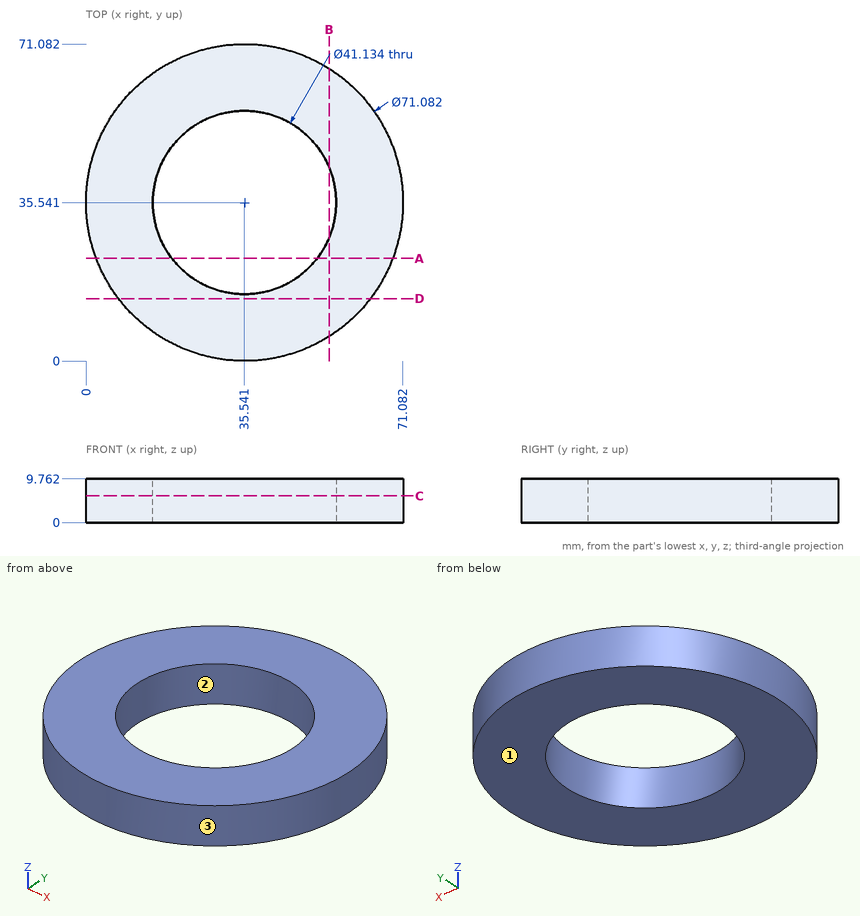
Here's the drawing with two shaded views (mm, measured from the low corner). I have some questions. Coordinates: 2 decimals unless noted, no trailing zeros. Loops run counter-clockwise (first coordinate to the right, second up) from the corner with the lowest first, then second, coordinate; pieces in that order, holes last. Notation, with made-up numbers: M 38.25,31 L 48.25,31 A21 ccw 48.25,41 Z; hole C -25.5,-14.75 d2. An arc over 180 degrees is marked long. Answer as CSV lines item,"result". Start each with the question number.
1. Suppose I cut it at A-A, the plane y = 23. List the corners of the cut face in (x, z) for me, plus the area to 3 significant figures.
2. Suppose I cut it at B-B, the plane x = 54.5. List the corners of the cut face in (y, z) for me (1 decimal).
3. For pin 1 Ø1.5 at (y, z) = (44, 8.5) entering from -X; pin 2 Ø5 at (x, z) = (36.5, 8) entering from -Y; pin 3 Ø1.5 at (x, z) = (38.5, 5.5) entering from -Y, each with a flat end and sliding along its axis, tell me the tip position at first contact or that it passes through.
4. If I drill on probe 1 along X at (y, z) = (35.5, 9.25) (1 decimal); probe 2 along X at (y, z) = (53, 6) (1 decimal), over which ranges is the centre line in solid material (lowest first)? Write a range as [from, to].
5. Suppose I cut it at D-D, the plane y = 14. List the corners of the cut face in (x, z) for me, plus the area to 3 significant figures.
6. Thinking about a two-plate mould opening in X: for the marked faces 1, 2 and 3, which applies, +X half, -X half, draft (parallel to the pull), parting line (faces both ways), or undercut?
7. Suppose I cut it at C-C, the plane z = 6. List the corners of the cut face in (x, y) for me (1 decimal), plus the area to 3 significant figures.
Output:
1,outline,"M 2.29,0 L 19.24,0 L 19.24,9.76 L 2.29,9.76 Z; M 51.84,0 L 68.8,0 L 68.8,9.76 L 51.84,9.76 Z"
1,area,"331 mm^2"
2,outline,"M 5.5,0 L 27.6,0 L 27.6,9.8 L 5.5,9.8 Z; M 43.5,0 L 65.6,0 L 65.6,9.8 L 43.5,9.8 Z"
3,pin 1,"stops at x = 0.85"
3,pin 2,"stops at y = 0"
3,pin 3,"stops at y = 0.07"
4,probe 1,"x = [0, 15], [56.1, 71.1]"
4,probe 2,"x = [4.6, 24.7], [46.4, 66.5]"
5,outline,"M 7.27,0 L 63.81,0 L 63.81,9.76 L 7.27,9.76 Z"
5,area,"552 mm^2"
6,face 1,"draft"
6,face 2,"undercut"
6,face 3,"parting line"
7,outline,"C 35.5,35.5 d71.1; hole C 35.5,35.5 d41.1"
7,area,"2,640 mm^2"
